from build123d import *

# Parameters (mm, degrees)
F0_W      = 151.9949287176
F0_H      = 151.8344208598
F1_DEPTH  = 25.4
F2_DEPTH  = 25.4
F3_W      = 151.9949287176
F3_H      = 151.8344208598
F4_DEPTH  = 25.4
F5_DEPTH  = 25.4
F6_W      = 151.9949287176
F6_H      = 151.8344208598
F7_DEPTH  = 25.4
F9_DEPTH  = 25.4
F10_W     = 151.9949287176
F10_H     = 127
F11_DEPTH = 25.4
F12_W     = 151.9949287176
F12_H     = 127
F13_DEPTH = 25.4
F15_DEPTH = 25.4
F16_W     = 202.6344208598
F16_H     = 127
F17_DEPTH = 25.4
F18_W     = 202.6344208598
F18_H     = 127
F19_DEPTH = 25.4
F21_DEPTH = 25.4
F22_DEPTH = 25.4


with BuildPart() as f1:
    # F0 (on Top) → F1 (new body)
    with BuildSketch(Plane.XY):
        with Locations((0, 0.2407543361)):
            Rectangle(F0_W, F0_H)
    extrude(amount=F1_DEPTH)

    # F2 (add): a face of the model
    f2_faces = [f1.faces().sort_by_distance(p)[0] for p in [
        (0, 0.2407543361, 25.4),
    ]]
    extrude(f2_faces, amount=F2_DEPTH)

    # F3 (on face) → F4 (join)
    with BuildSketch(Plane.XY.offset(50.8)):
        with Locations((0, 0.2407543361)):
            Rectangle(F3_W, F3_H)
        Polygon((-54.7822974622, -60.2384917438), (-54.3631203473, -51.7334751785), (-54.3631203473, 43.2750284672), (20.9696162492, -43.1563518941), (29.0977004915, -51.7212189734), (30.7523328811, 43.9543314278), (45.7475273532, 43.6950014908), (45.7475273532, -59.0233169496), (20.4021297395, -59.0233169496), (-46.2220385671, 21.2365556508), (-46.2220385671, -60.2384917438), align=None, mode=Mode.SUBTRACT)
    extrude(amount=F4_DEPTH)

    # F5 (add): a face of the model
    f5_faces = [f1.faces().sort_by_distance(p)[0] for p in [
        (0, 0.2407543361, 0),
    ]]
    extrude(f5_faces, amount=F5_DEPTH)

    # F6 (on face) → F7 (join)
    with BuildSketch(Plane(origin=(0, 0, -25.4), x_dir=(1, 0, 0), z_dir=(0, 0, -1))):
        with Locations((0, -0.2407543361)):
            Rectangle(F6_W, F6_H)
        Polygon((-46.6125570238, -64.9226754904), (-59.8847456276, -64.9226754904), (-17.829503864, 58.8444620371), (4.2375051416, 58.8444620371), (56.6866248846, -65.7222047448), (40.2163229883, -65.7222047448), (19.2686561495, -24.6263965964), (-34.2998057604, -24.6263965964), align=None, mode=Mode.SUBTRACT)
    extrude(amount=F7_DEPTH)

    # F8 (on face) → F9 (join)
    with BuildSketch(Plane(origin=(0, 0, -25.4), x_dir=(1, 0, 0), z_dir=(0, 0, -1))):
        Polygon((13.0323283374, -4.5461022683), (-8.3950581029, 51.8086031079), (-27.544008353, -4.5461022683), align=None)
    extrude(amount=F9_DEPTH)

    # F10 (on face) → F11 (join)
    with BuildSketch(Plane.XZ.offset(75.6764560938)):
        with Locations((0, 12.7)):
            Rectangle(F10_W, F10_H)
        Polygon((-45.7281582057, -43.2857945561), (-45.261003077, -35.732280463), (-45.261003077, 60.8546175063), (16.7235676199, -32.2795137763), (16.7235676199, 63.9280602336), (28.3728465438, 63.9280602336), (28.3728465438, -41.1987639964), (3.2877130434, -41.1987639964), (-37.5465713441, 31.0532525182), (-37.5465713441, -43.2857945561), align=None, mode=Mode.SUBTRACT)
    extrude(amount=F11_DEPTH)

    # F12 (on face) → F13 (join)
    with BuildSketch(Plane(origin=(0, 76.157964766, 0), x_dir=(-1, 0, 0), z_dir=(0, 1, 0))):
        with Locations((0, 12.7)):
            Rectangle(F12_W, F12_H)
        Polygon((-41.00927338, -34.1472737491), (-51.6761131585, -33.7340943515), (-18.3558836579, 56.9384694099), (3.0622561462, 59.0705610812), (53.1387478113, -36.8585251272), (38.4384579957, -36.8585251272), (18.0476587266, 0.3876684059), (-25.5533028394, 0.3876684059), align=None, mode=Mode.SUBTRACT)
    extrude(amount=F13_DEPTH)

    # F14 (on face) → F15 (join)
    with BuildSketch(Plane(origin=(0, 76.157964766, 0), x_dir=(-1, 0, 0), z_dir=(0, 1, 0))):
        Polygon((-7.2864516565, 50.0721470643), (-17.2580555081, 22.9369532317), (1.9618875813, 23.7948019058), align=None)
    extrude(amount=F15_DEPTH)

    # F16 (on face) → F17 (join)
    with BuildSketch(Plane.YZ.offset(75.9974643588)):
        with Locations((0.2407543361, 12.7)):
            Rectangle(F16_W, F16_H)
        Polygon((-57.3391616344, -46.8861833215), (-56.8041577935, -32.4410460889), (-56.8041577935, 55.5672757328), (-1.4311361592, -33.7785594165), (-1.4311361592, 56.6372871399), (10.4727260768, 56.6372871399), (10.4727260768, 55.9685304761), (10.4727260768, -45.8161756396), (-11.8637345731, -45.8161756396), (-51.0528497398, 30.823295936), (-51.0528497398, -46.8861833215), align=None, mode=Mode.SUBTRACT)
    extrude(amount=F17_DEPTH)

    # F18 (on face) → F19 (join)
    with BuildSketch(Plane(origin=(-75.9974643588, 0, 0), x_dir=(0, -1, 0), z_dir=(-1, 0, 0))):
        with Locations((-0.2407543361, 12.7)):
            Rectangle(F18_W, F18_H)
        Polygon((-44.0442897379, -38.8611070812), (-55.2793927491, -38.8611070812), (-25.1853633672, 62.5223442912), (-3.3839091193, 62.5223442912), (45.1677963138, -40.5998714268), (30.7226609439, -40.5998714268), (7.8511973843, 4.6080499887), (-30.5354129523, 4.6080499887), align=None, mode=Mode.SUBTRACT)
    extrude(amount=F19_DEPTH)

    # F20 (on face) → F21 (join)
    with BuildSketch(Plane(origin=(-75.9974643588, 0, 0), x_dir=(0, -1, 0), z_dir=(-1, 0, 0))):
        Polygon((-14.065767224, 48.3413906964), (-23.1149289757, 17.8557671607), (-5.3965207189, 18.1462336332), align=None)
    extrude(amount=F21_DEPTH)

    # F22 (add): a face of the model
    f22_faces = [f1.faces().sort_by_distance(p)[0] for p in [
        (33.0748285463, -57.5754775221, 50.8),
    ]]
    extrude(f22_faces, amount=F22_DEPTH)


solid = f1.part
Geometry check sheet. Reference: the model listing, model coordinates, mm. A direction names the side the tool comes from. Give positions to 0.01 mm unless a question says otherwise; leave off trailing zeros. Order: outer loops, then holes, each group sorted by start corner. A loop starts at its lowest first (then second) coordinate and runs counter-clockwise, first axis right, second up.
1. Scan lines: line 1 (Y direction, x = 93.5, z = 38); line 2 (X direction, y = 86.5, z = 36.5); line 3 (X direction, y = 90, z = -6). Record each from-to range of solid material in increasing order.
Completed:
line 1: y = -101.08 to -56.8, -45.92 to -1.43, 10.47 to 101.56
line 2: x = -101.4 to -14.84, 2.51 to 12.27, 25.87 to 101.4
line 3: x = -101.4 to -37.03, -21.54 to 28.41, 41.48 to 101.4
2. Draft check along Y on faces 1 (the face through (8, 101.558, 31)), 2 (the face through (-42, -88, -43.286)), 3 (the face through (-75.997, 12, 15)). Enter one of: pulls with the +Y half, pulls with the -Y half, needs draft (parallel to the pull), parting line crosses it, or undercut.
Completed:
face 1: pulls with the +Y half
face 2: needs draft
face 3: undercut
3. Access from +Z, -Z, +X, -X, +Y, -Y to the whole of each face (thin tool, end or side, straight path). Record for faces 4 (the face through (7.78, 88.68, 23.36)), 5 (the face through (-40.37, 44.49, -37.92)), 6 (the face through (-8, -18, -50.8)), 7 (the face through (-88.52, 9.67, 33.03)), 8 (the face through (89, -1, -45.816)).
Completed:
face 4: +Y
face 5: -Z
face 6: -Z, +X, -X, +Y, -Y
face 7: -X
face 8: +X
4. Sectioned sample at A-A (x = -84). Record the boundary of the cut face in (y, z).
Completed:
outline: (-101.08, -50.8) - (101.56, -50.8) - (101.56, 76.2) - (-101.08, 76.2) - close; (5.4, 18.15) - (23.11, 17.86) - (14.07, 48.34) - close; hole (-45.17, -40.6) - (-30.72, -40.6) - (-7.85, 4.61) - (30.54, 4.61) - (44.04, -38.86) - (55.28, -38.86) - (25.19, 62.52) - (3.38, 62.52) - close
5. Sectioned sample at D-D (x = 34). Record the boundary of the cut face in (y, z), then the cut area to 3 significant figures.
Completed:
outline: (-101.08, -50.8) - (11.84, -50.8) - (11.84, -25.4) - (53.53, -25.4) - (53.53, -50.8) - (101.56, -50.8) - (101.56, -18.49) - (76.16, -18.49) - (76.16, 14.37) - (101.56, 14.37) - (101.56, 76.2) - (-101.08, 76.2) - close
area: 23,800 mm2
6. Sectioned sample at C-C (x = -23). Record the boundary of the cut face in (y, z).
Completed:
outline: (-101.08, -50.8) - (-43.63, -50.8) - (-43.63, -25.4) - (-8.83, -25.4) - (-8.83, -50.8) - (4.55, -50.8) - (4.55, -25.4) - (24.63, -25.4) - (24.63, -50.8) - (101.56, -50.8) - (101.56, -8.66) - (76.16, -8.66) - (76.16, 20.88) - (101.56, 20.88) - (101.56, 76.2) - (-101.08, 76.2) - (-101.08, 27.41) - (-75.68, 27.41) - (-75.68, 5.31) - (-101.08, 5.31) - close
7. Sectioned sample at B-B (y = -19). Record the boundary of the cut face in (x, z), then the cut area to 3 significant figures.
Completed:
outline: (-101.4, -50.8) - (-31.37, -50.8) - (-31.37, -25.4) - (-19.54, -25.4) - (-19.54, -50.8) - (4.08, -50.8) - (4.08, -25.4) - (21.01, -25.4) - (21.01, -50.8) - (101.4, -50.8) - (101.4, -31.86) - (76, -31.86) - (76, -5.43) - (101.4, -5.43) - (101.4, 76.2) - (-101.4, 76.2) - (-101.4, 14.98) - (-76, 14.98) - (-76, -17.43) - (-101.4, -17.43) - close
area: 23,500 mm2
